Build history of the part. All positions in model axes, mm. A direction names the side the tool comes from. Coordinates: 2 decimals unless noted, no trailing zeros. Order: outer loops, then holes, each group sorted by start corner. A loop starts at its lowest first (then second) coordinate and runs counter-clockwise, first axis right, second up. Notation, with made-up numbers: M -4.5,12.25 L 47.5,12.25 A17 ccw 47.5,23.25 Z; hole C -10,-0.5 d3. An arc over 180 degrees is marked long. Use a Markdown table: item, result. Add a question column.
from build123d import *

# Parameters (mm, degrees)
SKETCH_1_R               = 13.1
EXTRUDE_1_DEPTH          = 30
CUT_EXTRUDE_1_DEPTH      = 31
CUT_EXTRUDE_1_DEPTH_BACK = 31
CUT_EXTRUDE_2_DEPTH      = 31
CUT_EXTRUDE_2_DEPTH_BACK = 31
CUT_EXTRUDE_3_DEPTH      = 4
CUT_EXTRUDE_3_DEPTH_BACK = 4
SKETCH_4_R               = 3.5
CUT_EXTRUDE_4_DEPTH      = 4
CUT_EXTRUDE_4_DEPTH_BACK = 4
SKETCH_5_R               = 3.5


with BuildPart() as part:
    # Sketch 1 → Extrude 1 (new body)
    with BuildSketch(Plane(origin=(0, 0, 0), x_dir=(0, 0, -1), z_dir=(1, 0, 0))):
        with BuildLine():
            Line((-31, 0), (31, 0))
            Line((31, 0), (31, 4))
            Line((31, 4), (16.527117977, 49.902117399))
            ThreePointArc((16.527117977, 49.902117399), (15.43989607, 51.419333813), (13.665967125, 52))
            Line((13.665967125, 52), (-13.665967125, 52))
            ThreePointArc((-13.665967125, 52), (-15.43989607, 51.419333813), (-16.527117977, 49.902117399))
            Line((-16.527117977, 49.902117399), (-31, 4))
            Line((-31, 4), (-31, 0))
        make_face()
        with Locations((0, 33)):
            Circle(SKETCH_1_R, mode=Mode.SUBTRACT)
    extrude(amount=EXTRUDE_1_DEPTH)

    # Sketch 2 → Cut-Extrude 1 (cut, two sides: drawn at the far end of the back side and taken through both)
    with BuildSketch(Plane.XY.offset(-CUT_EXTRUDE_1_DEPTH_BACK)):
        with BuildLine():
            Line((5, 4), (30, 4))
            Line((30, 4), (30, 52))
            Line((30, 52), (4, 52))
            Line((4, 52), (4, 5))
            ThreePointArc((4, 5), (4.292893219, 4.292893219), (5, 4))
        make_face()
    extrude(amount=CUT_EXTRUDE_1_DEPTH + CUT_EXTRUDE_1_DEPTH_BACK, mode=Mode.SUBTRACT)

    # Sketch 3 → Cut-Extrude 2 (cut, two sides: drawn at the far end of the back side and taken through both)
    with BuildSketch(Plane.XY.offset(-CUT_EXTRUDE_2_DEPTH_BACK)):
        with BuildLine():
            Line((-1, -1), (1.5, -1))
            Line((1.5, -1), (1.5, 0))
            ThreePointArc((1.5, 0), (0.439339828, 0.439339828), (0, 1.5))
            Line((0, 1.5), (-1, 1.5))
            Line((-1, 1.5), (-1, -1))
        make_face()
    extrude(amount=CUT_EXTRUDE_2_DEPTH + CUT_EXTRUDE_2_DEPTH_BACK, mode=Mode.SUBTRACT)

    # Sketch 4 → Cut-Extrude 3 (cut, two sides: drawn at the far end of the back side and taken through both)
    with BuildSketch(Plane(origin=(0, 0, 0), x_dir=(1, 0, 0), z_dir=(0, 1, 0)).offset(-CUT_EXTRUDE_3_DEPTH_BACK)):
        with Locations(Location((23, 23, 0), (0, 0, 270))):
            Circle(SKETCH_4_R)
    extrude(amount=CUT_EXTRUDE_3_DEPTH + CUT_EXTRUDE_3_DEPTH_BACK, mode=Mode.SUBTRACT)

    # Sketch 5 → Cut-Extrude 4 (cut, two sides: drawn at the far end of the back side and taken through both)
    with BuildSketch(Plane(origin=(0, 0, 0), x_dir=(1, 0, 0), z_dir=(0, 1, 0)).offset(-CUT_EXTRUDE_4_DEPTH_BACK)):
        with Locations(Location((23, -23, 0), (0, 0, 270))):
            Circle(SKETCH_5_R)
    extrude(amount=CUT_EXTRUDE_4_DEPTH + CUT_EXTRUDE_4_DEPTH_BACK, mode=Mode.SUBTRACT)


solid = part.part
(1) Which spindle directions (+Z, -Z, +X, -X, +Y, -Y) get a long thin tool onto all of the face, cutting with end or side? Do faces 5 (the flat face through (16, 0, 0)), 6 (the flat face through (17, 4, 0)). Say none if no direction does.
(2) Mould opens along Z. For faces 1 (the cylindrical face through (1.972, 45.989, 1.705)), 2 (the flat face through (4, 18, 0)), 3 (the cylindrical face through (25.95, 1.97, -21.12)), 4 (the cylindrical face through (1.972, 51.435, 15.418)) say: released by +Z, released by -Z, zero draft, split by the parting line, or undercut.
(3) Slice it at D-D on x = 18.75. Give the cut face in (y, z), and give its area (3 significant figures).
(4) Drill centre lines: line 1 along Z through (x, y) = (23, 1.4); line 2 along Y through (x, z) = (19.5, -19). Where is each one in solid material? Low to high. Write a range as from..to.
(5) Drop flat-ended pins along their axis: P1, Ø4, axis at x = 5, y = 41, coming from the +Z side; P2, Ø14, axis at y = 36.5, z = 4.5, coming from the +X side; P3, Ø11, axis at x = 23, z = -23, coming from the +Y side; P4, Ø2, axis at y = 5.5, z = 3.5, coming from the +X side. Give the stop position or say it passes through.
(6) Slice it at A-A on z = 0. Give the cut face in (x, y).
(7) Slice it at B-B on y = 33. Give the cut face in (x, z), and give its area (3 significant figures).
(8) Slice it at C-C on y = 24. Give the cut face in (x, z).
Solutions:
| question | item | result |
|---|---|---|
| 1 | face 5 | +Z, -Z, +X, -X, -Y |
| 1 | face 6 | +Z, -Z, +X, +Y |
| 2 | face 1 | undercut |
| 2 | face 2 | zero draft |
| 2 | face 3 | undercut |
| 2 | face 4 | released by +Z |
| 3 | outline | M 0,-31 L 4,-31 L 4,31 L 0,31 Z |
| 3 | area | 248 mm² |
| 4 | line 1 | -31..-26.5, -19.5..19.5, 26.5..31 |
| 4 | line 2 | 0..4 |
| 5 | P1 | z = 19.88 |
| 5 | P2 | through |
| 5 | P3 | y = 4 |
| 5 | P4 | x = 4.13 |
| 6 | outline | M 0,1.5 A1.5 ccw 1.5,0 L 30,0 L 30,4 L 5,4 A1 cw 4,5 L 4,19.9 L 0,19.9 Z; M 0,46.1 L 4,46.1 L 4,52 L 0,52 Z |
| 7 | outline | M 0,-21.86 L 4,-21.86 L 4,-13.1 L 0,-13.1 Z; M 0,13.1 L 4,13.1 L 4,21.86 L 0,21.86 Z |
| 7 | area | 70.1 mm² |
| 8 | outline | M 0,-24.69 L 4,-24.69 L 4,-9.52 L 0,-9.52 Z; M 0,9.52 L 4,9.52 L 4,24.69 L 0,24.69 Z |
